The drawing under review shows one solid part. Ordinate dimensions are in mm from its lowest x, y, z. A direction names the side the tool comes from. Coordinates: 2 decimals unless noted, no trailing zeros. Loops run counter-clockwise (first coordinate to the right, second up) from the corner with the lowest first, then second, coordinate; pieces in that order, holes last. Notation, with made-up numbers: (41, 7) - (54, 7) arc R34 ccw to (54, 37) - close; hole circle Ø7 at (37.25, -36). An arc over 180 degrees is marked (long way). Use one line per item in the form item = value. Start each with the question number.
1. Add section B-B on y = 22.5. Give the boundary of the cut face in (x, z) (3 decimals), and give its area (3 significant figures).
2. Machinability: for the marked faces 4, 5 and 6, which of the approach directions +Z, -Z, +X, -X, +Y, -Y give a long, thin tool a straight path to every point of the face, cutting with its end or side? Answer none if there is none.
3. Draft analysis for pull direction Y (two halves, no side actions). For the marked faces 1, 2 and 3, state which applies: +Y half, -Y half, draft (parallel to the pull), parting line (faces both ways), or undercut.
4. For pin 1 Ø1.6 at (x, y) = (1.5, 43.5) entering from -Z; pin 2 Ø1.6 at (x, y) = (36.5, 36.5) entering from -Z; pin 3 Ø3.5 at (x, y) = (8.5, 36.5) entering from -Z, all flat-tipped, find the tip position at first contact; note any pin that passes through.
5. Add section A-A on z = 4.5. Give the boundary of the cut face in (x, y) (3 decimals), and give its area (4 significant figures).
6. Add section D-D on y = 36.5. Give the boundary of the cut face in (x, z) (3 decimals).
7. To check wall thickness, follow probe 1 along X at (y, z) = (1.5, 2.25) (3 decimals); probe 2 along Y at (x, z) = (8.5, 11) (3 decimals). State the ranges of each line that lie inside material, in increasing order.
8. Add section C-C on x = 17. Give the boundary of the cut face in (y, z), and give its area (3 significant figures).
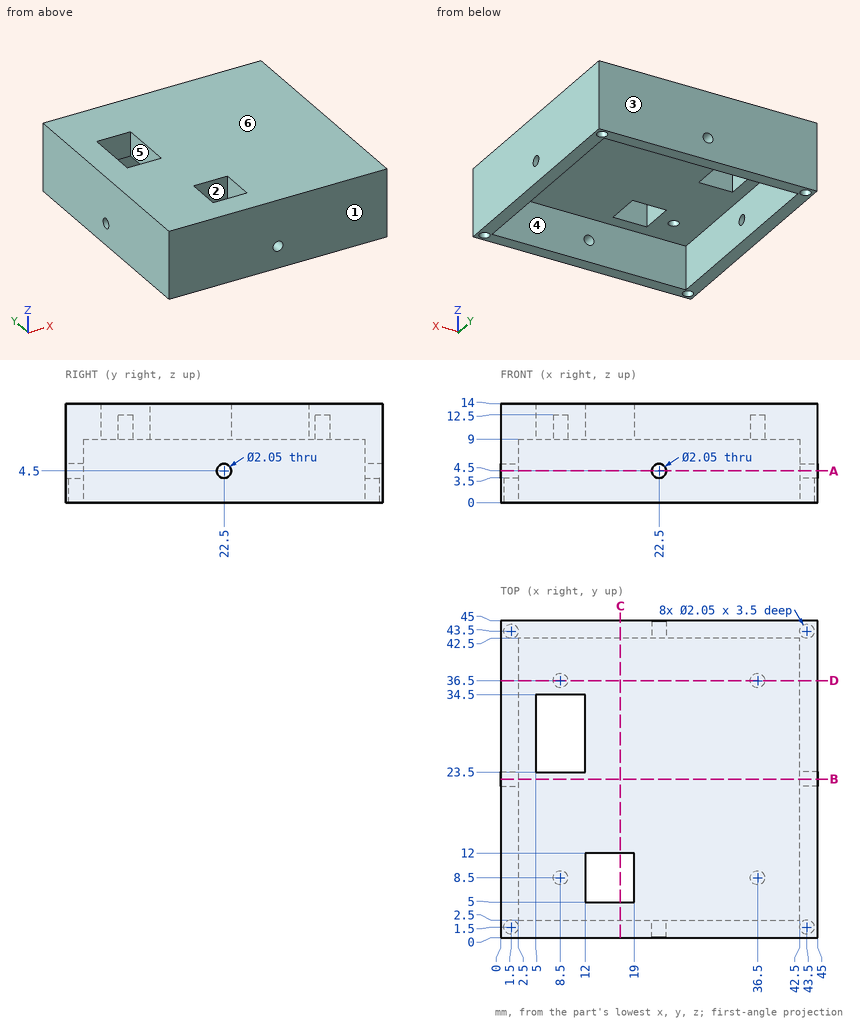
Conclusion:
q1.outline = (0, 0) - (2.5, 0) - (2.5, 3.475) - (0, 3.475) - close; (0, 5.525) - (2.5, 5.525) - (2.5, 9) - (42.5, 9) - (42.5, 5.525) - (45, 5.525) - (45, 14) - (0, 14) - close; (42.5, 0) - (45, 0) - (45, 3.475) - (42.5, 3.475) - close
q1.area = 260 mm^2
q2.face_4 = -Z
q2.face_5 = +Z, -Z
q2.face_6 = +Z, +X, -X, +Y, -Y
q3.face_1 = -Y half
q3.face_2 = undercut
q3.face_3 = +Y half
q4.pin_1 = 3.5
q4.pin_2 = 12.5
q4.pin_3 = 9
q5.outline = (0, 0) - (21.475, 0) - (21.475, 2.5) - (2.5, 2.5) - (2.5, 21.475) - (0, 21.475) - close; (0, 23.525) - (2.5, 23.525) - (2.5, 42.5) - (21.475, 42.5) - (21.475, 45) - (0, 45) - close; (23.525, 0) - (45, 0) - (45, 21.475) - (42.5, 21.475) - (42.5, 2.5) - (23.525, 2.5) - close; (23.525, 42.5) - (42.5, 42.5) - (42.5, 23.525) - (45, 23.525) - (45, 45) - (23.525, 45) - close
q5.area = 404.5 mm^2
q6.outline = (0, 0) - (2.5, 0) - (2.5, 9) - (7.475, 9) - (7.475, 12.5) - (9.525, 12.5) - (9.525, 9) - (35.475, 9) - (35.475, 12.5) - (37.525, 12.5) - (37.525, 9) - (42.5, 9) - (42.5, 0) - (45, 0) - (45, 14) - (0, 14) - close
q7.probe_1 = 0 to 0.475, 2.525 to 42.475, 44.525 to 45
q7.probe_2 = 0 to 7.475, 9.525 to 23.5, 34.5 to 35.475, 37.525 to 45
q8.outline = (0, 0) - (2.5, 0) - (2.5, 9) - (5, 9) - (5, 14) - (0, 14) - close; (12, 9) - (42.5, 9) - (42.5, 0) - (45, 0) - (45, 14) - (12, 14) - close
q8.area = 235 mm^2
